Autodesk Inventor part; units mm, degrees
ref_plane "YZ Plane" through (0, 0, 0) normal (1, 0, 0) x (0, 1, 0)
ref_plane "XZ Plane" through (0, 0, 0) normal (0, 1, 0) x (-1, 0, 0)
ref_plane "XY Plane" through (0, 0, 0) normal (0, 0, 1) x (1, 0, 0)
sketch "Sketch1" plane through (0, 0, 0) normal (0, 0, 1) x (1, 0, 0)
  line L0 (-12.7, -12.7) -> (12.7, -12.7)
  line L1 (12.7, -12.7) -> (12.7, 12.7)
  line L2 (12.7, 12.7) -> (-12.7, 12.7)
  line L3 (-12.7, 12.7) -> (-12.7, -12.7)
  line L4 (-12.7, -12.7) -> (12.7, 12.7) construction
  line L5 (12.7, -12.7) -> (-12.7, 12.7) construction
  line L6 (11.1125, -11.1125) -> (-11.1125, -11.1125)
  line L7 (-11.1125, -11.1125) -> (-11.1125, 11.1125)
  line L8 (-11.1125, 11.1125) -> (11.1125, 11.1125)
  line L9 (11.1125, 11.1125) -> (11.1125, -11.1125)
  line L10 (11.1125, -11.1125) -> (-11.1125, 11.1125) construction
  line L11 (-11.1125, -11.1125) -> (11.1125, 11.1125) construction
  point P0 (0, 0)
  dimension "d0" = 25.4
  dimension "d1" = 25.4
  dimension "d3" = 22.225
  dimension "d4" = 22.225
extrude "Extrusion1" add sketch "Sketch1" along normal mid plane 88.9
sketch "Sketch2" plane through (-12.7, 12.7, 44.45) normal (0, 1, 0) x (1, 0, 0)
  line L0 (25.4, 0) -> (0, 0)
  point P0 (12.7, 44.45)
  point P1 (12.7, 6.35)
  point P2 (12.7, 31.75)
  point P3 (12.7, 57.15)
  point P4 (12.7, 0)
  point P5 (12.7, 0)
  dimension "d7" = 6.35
  dimension "d8" = 25.4
  dimension "d9" = 25.4
hole "Hole1" at (0, 12.7, 38.1) at (0, 12.7, 12.7) at (0, 12.7, -12.7) direction (0, -1, 0) diameter 5.1054 end through all
properties part number "DB1-006" material "Aluminum 6061"
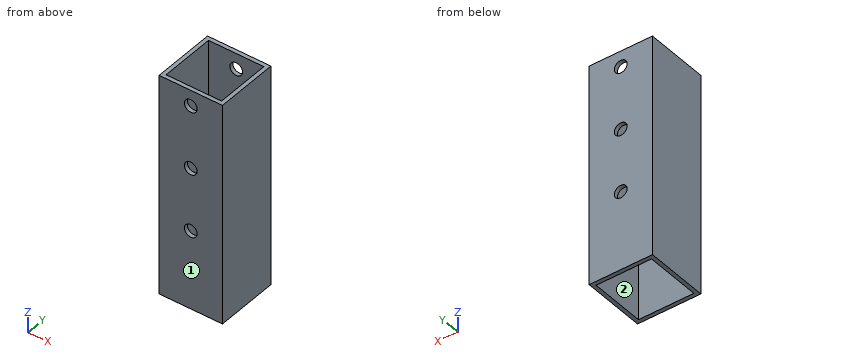
Could you check a few things on this model? Use its own coordinates, in mm. Face numbers are marked on the shaded views. A direction names the side the tool comes from. Round coordinates to 2 decimals unless told otherwise and drop trailing zeros. Loops run counter-clockwise (first coordinate to the right, second up) from the corner with the lowest first, then second, coordinate; pieces in that order, holes last. Notation, with made-up numbers: (-20.75, -32) -> (-15.75, -32) arc R19 ccw to (-15.75, -22) -> close; hole circle Ø9 at (60, 9). An arc over 180 degrees is marked (long way). One line per question, with ' | ' between items.
(1) If we section it at A-A on x = -5.5: List the corners of the cut face in (y, z) for me.
Model answer:
outline: (-12.7, -44.45) -> (-11.11, -44.45) -> (-11.11, 44.45) -> (-12.7, 44.45) -> close; (11.11, -44.45) -> (12.7, -44.45) -> (12.7, 44.45) -> (11.11, 44.45) -> close
(2) If we section it at C-C on z = -12.7: List the corners of the cut face in (x, y) for me.
Model answer:
outline: (-12.7, -12.7) -> (-2.55, -12.7) -> (-2.55, -11.11) -> (-11.11, -11.11) -> (-11.11, 11.11) -> (-2.55, 11.11) -> (-2.55, 12.7) -> (-12.7, 12.7) -> close; (2.55, -12.7) -> (12.7, -12.7) -> (12.7, 12.7) -> (2.55, 12.7) -> (2.55, 11.11) -> (11.11, 11.11) -> (11.11, -11.11) -> (2.55, -11.11) -> close
(3) For the marked faces 1 and 2, which set-ups out of +Z, -Z, +X, -X, +Y, -Y let a thin tool reach every point of the face, with its end or its side?
Model answer:
face 1: +Z, -Z, +X, -X, -Y | face 2: +Z, -Z
(4) If I drill on probe 1 along Z at (x, y) = (0, -11.9); probe 2 along X at (y, z) = (-6.25, -31.5), over which ranges is the centre line in solid material (lowest first)?
Model answer:
probe 1: z = -44.45 to -15.25, -10.15 to 10.15, 15.25 to 35.55, 40.65 to 44.45 | probe 2: x = -12.7 to -11.11, 11.11 to 12.7
(5) For pin 1 Ø4 at (x, z) = (0, 38.1) entering from -Y, with a flat end and sliding along its axis, tell me the tip position at first contact or that it passes through.
Model answer:
pin 1: passes through
(6) If we section it at D-D on x = 0: Count the separate pieces of the cut face and the enclosed holes in it, and give its area (3 significant figures).
Model answer:
separate pieces: 8 | enclosed holes: 0 | area: 234 mm^2
